Check sheet for the modelled part. Datum: model origin and axes. Units: mm. A direction names the side the tool comes from. Round coordinates to 2 decimals unless told otherwise and drop trailing zeros. Loops run counter-clockwise (first coordinate to the right, second up) from the corner with the lowest first, then second, coordinate; pieces in that order, holes last. Notation, with made-up numbers: M -26.5,-4.75 L -9.5,-4.75 A11 cw -9.5,7.25 Z; hole C 70.25,80.25 d2. An arc over 180 degrees is marked long. Write item = value, one per line. Start each with the question number.
(1) Go/stop test with flat-tipped pins: P1, Ø1.8, axis at x = 32.44, y = 54.92, coming from the +Z side; P2, Ø3, axis at x = -34.5, z = -1, coming from the -Y side; P3, Ø0.8, axis at x = 27, z = -1, coming from the +Y side; P4, Ø2, axis at y = 56.5, z = -2, coming from the -X side. Record where each tip stops, or that it passes through.
(2) Cross-section at A-A on z = -1.75. Record the boundary of the cut face in (x, y), plus the area to 3 significant figures.
(3) Cross-section at B-B on y = 32.5. Record the boundary of the cut face in (x, z).
(4) Set-up check for faces 4 (the face through (32, -55, 0.5)), 5 (the face through (-30.457, -53, -1)), 6 (the face through (36.443, 55, -1)), 7 (the face through (32.443, -59, -1)), 8 (the face through (31, 51.924, -1)): record each of +Z, -Z, +X, -X, +Y, -Y from which the full face is reachable in a straight line by a thin tool's end or side.
(5) Scan lines: L1, parallel to Y at x = 30, z = -0.65; L2, parallel to X at y = 52.5, z = -1.1; L3, parallel to Y at x = -9, z = -1.05. Record each from-to range of solid material in increasing order. Write a range as from..to.
(6) Mould release check, pull along Y, two halves, no side actions. Record for faces 1 (the face through (-1, -60.576, 0)), 2 (the face through (-31.75, 55.67, -1.02)), 3 (the face through (-36.557, 55, -1)): pulls with the +Y half, pulls with the -Y half, needs draft (parallel to the pull), parting line crosses it, or undercut.
(7) Cross-section at C-C on x = 14.5. Record the boundary of the cut face in (y, z).
from build123d import *

# Parameters (mm, degrees)
F5_DEPTH       = 2.5
F3_W           = 10
F3_H           = 7
F3_W_2         = 6.1
F3_H_2         = 9.5
F7_DEPTH       = 5
F8_D           = 2.2
F8_DEPTH       = 10
F8_CBORE_D     = 3.9
F8_CBORE_DEPTH = 2
F8_TIP         = 0.6609466809
F6_W           = 65
F6_H           = 3
F9_DEPTH       = 5


with BuildPart() as f5:
    # F0 (on Top) → F5 (new body)
    with BuildSketch(Plane.XY):
        with BuildLine():
            Line((32.4426109495, 61.9244772196), (-32.5573890505, 61.9244772196))
            ThreePointArc((-32.5573890505, 61.9244772196), (-37.5071365188, 59.8742246879), (-39.5573890505, 54.9244772196))
            Line((-39.5573890505, 54.9244772196), (-39.5573890505, -53.5755227804))
            ThreePointArc((-39.5573890505, -53.5755227804), (-37.5071365188, -58.5252702487), (-32.5573890505, -60.5755227804))
            Line((-32.5573890505, -60.5755227804), (32.4426109495, -60.5755227804))
            ThreePointArc((32.4426109495, -60.5755227804), (37.3923584178, -58.5252702487), (39.4426109495, -53.5755227804))
            Line((39.4426109495, -53.5755227804), (39.4426109495, 54.9244772196))
            ThreePointArc((39.4426109495, 54.9244772196), (37.3923584178, 59.8742246879), (32.4426109495, 61.9244772196))
        make_face()
        with BuildLine():
            ThreePointArc((-36.5573890505, 54.9244772196), (-35.3858161753, 57.7529043443), (-32.5573890505, 58.9244772196))
            Line((-32.5573890505, 58.9244772196), (32.4426109495, 58.9244772196))
            ThreePointArc((32.4426109495, 58.9244772196), (35.2710380742, 57.7529043443), (36.4426109495, 54.9244772196))
            Line((36.4426109495, 54.9244772196), (36.4426109495, -53.5755227804))
            ThreePointArc((36.4426109495, -53.5755227804), (35.2710380742, -56.4039499052), (32.4426109495, -57.5755227804))
            Line((32.4426109495, -57.5755227804), (-32.5573890505, -57.5755227804))
            ThreePointArc((-32.5573890505, -57.5755227804), (-35.3858161753, -56.4039499052), (-36.5573890505, -53.5755227804))
            Line((-36.5573890505, -53.5755227804), (-36.5573890505, 54.9244772196))
        make_face(mode=Mode.SUBTRACT)
        with BuildLine():
            Line((32.4426109495, 58.9244772196), (-32.5573890505, 58.9244772196))
            ThreePointArc((-32.5573890505, 58.9244772196), (-35.3858161753, 57.7529043443), (-36.5573890505, 54.9244772196))
            Line((-36.5573890505, 54.9244772196), (-36.5573890505, -53.5755227804))
            ThreePointArc((-36.5573890505, -53.5755227804), (-35.3858161753, -56.4039499052), (-32.5573890505, -57.5755227804))
            Line((-32.5573890505, -57.5755227804), (32.4426109495, -57.5755227804))
            ThreePointArc((32.4426109495, -57.5755227804), (35.2710380742, -56.4039499052), (36.4426109495, -53.5755227804))
            Line((36.4426109495, -53.5755227804), (36.4426109495, 54.9244772196))
            ThreePointArc((36.4426109495, 54.9244772196), (35.2710380742, 57.7529043443), (32.4426109495, 58.9244772196))
        make_face()
    extrude(amount=F5_DEPTH)

    # F3 (on offset) → F7 (join)
    with BuildSketch(Plane.XY.offset(2.5)):
        with Locations((31.4426109495, 55.4244772196)):
            Rectangle(F3_W, F3_H)
        with Locations((-31.5573890505, 55.4244772196)):
            Rectangle(F3_W, F3_H)
        with Locations((-33.5073890505, -52.8255227804)):
            Rectangle(F3_W_2, F3_H_2)
        Polygon((36.4426109495, -57.5755227804), (36.4426109495, -48.0755227804), (20.3426109495, -48.0755227804), (22.4426109495, -57.5755227804), align=None)
    extrude(amount=-F7_DEPTH)

    # F8
    with Locations(Plane.XY.offset(2.5)):
        with Locations((-32.5573890505, 54.9244772196), (32.4426109495, 54.9244772196), (32.4426109495, -53.5755227804), (-32.5573890505, -53.5755227804)):
            CounterBoreHole(F8_D / 2, F8_CBORE_D / 2, F8_CBORE_DEPTH, depth=F8_DEPTH)
            with Locations((0, 0, -(F8_DEPTH + F8_TIP / 2))):  # 118° drill point
                Cone(0, F8_D / 2, F8_TIP, mode=Mode.SUBTRACT)

    # F6 (on offset) → F9 (join)
    with BuildSketch(Plane.XY.offset(2.5)):
        with Locations((-0.0573890505, -59.0755227804)):
            Rectangle(F6_W, F6_H)
    extrude(amount=-F9_DEPTH)


solid = f5.part
Result:
q1.P1 = through
q1.P2 = -60.53
q1.P3 = 58.92
q1.P4 = -36.56
q2.outline = M -36.56,-57.58 L -32.56,-57.58 L -32.56,-60.58 L 32.44,-60.58 L 32.44,-57.58 L 36.44,-57.58 L 36.44,-48.08 L 20.34,-48.08 L 22.44,-57.58 L -30.46,-57.58 L -30.46,-48.08 L -36.56,-48.08 Z; M -36.56,51.92 L -26.56,51.92 L -26.56,58.92 L -36.56,58.92 Z; M 26.44,51.92 L 36.44,51.92 L 36.44,58.92 L 26.44,58.92 Z; hole C -32.56,-53.58 d2.2; hole C -32.56,54.92 d2.2; hole C 32.44,-53.58 d2.2; hole C 32.44,54.92 d2.2
q2.area = 521 mm^2
q3.outline = M -39.56,0 L 39.44,0 L 39.44,2.5 L -39.56,2.5 Z
q4.face_4 = +Z
q4.face_5 = -Z
q4.face_6 = -Z, +X, +Y, -Y
q4.face_7 = -Z, +X, -Y
q4.face_8 = -Z, +X, -X
q5.L1 = -60.58..-48.08, 51.92..58.92
q5.L2 = -36.56..-26.56, 26.44..36.44
q5.L3 = -60.58..-57.58
q6.face_1 = pulls with the -Y half
q6.face_2 = undercut
q6.face_3 = needs draft
q7.outline = M -60.58,-2.5 L -57.58,-2.5 L -57.58,0 L 61.92,0 L 61.92,2.5 L -60.58,2.5 Z
